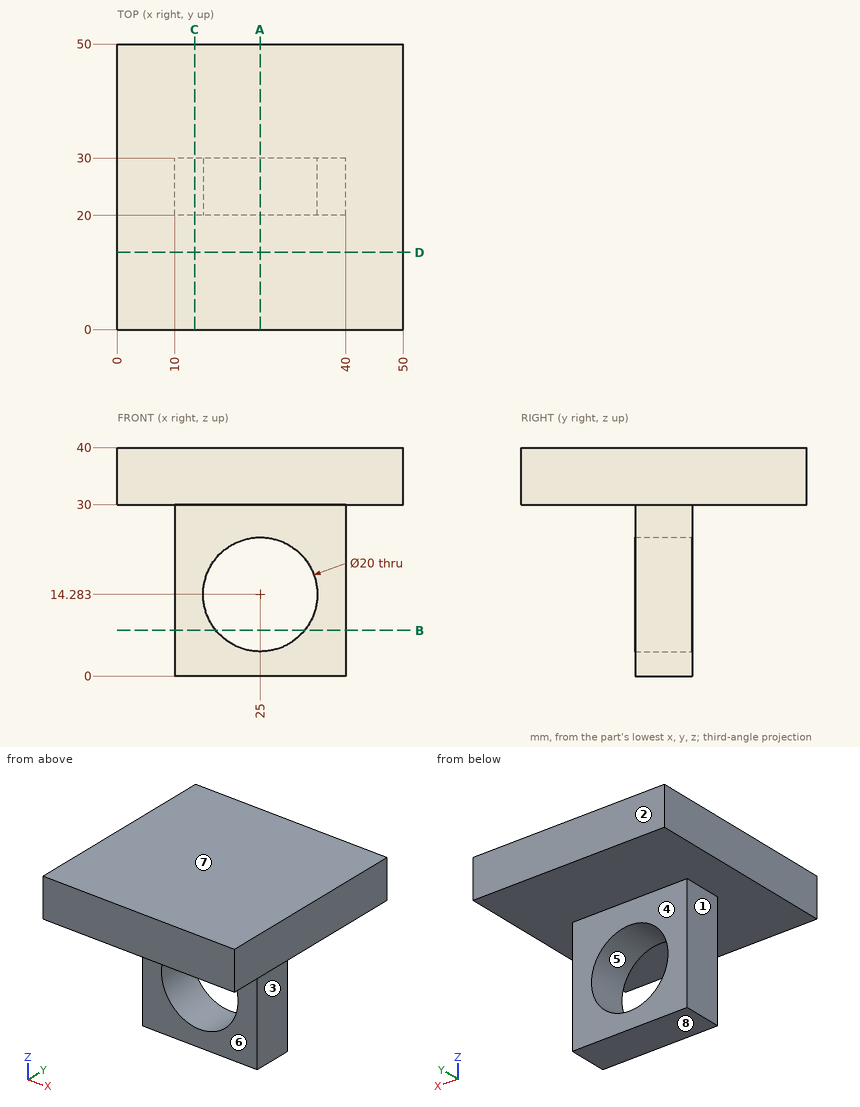
Verification items for this drawing (mm, ordinates from the low corner). A direction names the side the tool comes from. Round coordinates to 2 decimals unless told otherwise and drop trailing zeros. Write each loop counter-clockwise with the first axis right and the second up, starting at its lowest first coordinate (ties: lowest second). Pieces come first, ordered by that corner, then holes. Notation, with made-up numbers: M 3.25,73 L 28.25,73 A29 cw 28.25,97 Z; hole C 22.5,-39 d1. An arc over 180 degrees is marked long. Write item = value, one per line. Start each with the question number.
1. Section check C-C, the plane x = 13.5. Record the cut outline in (y, z).
2. Section check D-D, the plane y = 13.5. Record the cut outline in (x, z), then the cut area to 3 significant figures.
3. Scan lines: line 1 (Z direction, x = 25, y = 25.75); line 2 (Z direction, x = 4, y = 3.5); line 3 (Y direction, x = 37, z = 17.5). Record each from-to range of solid material in increasing order. Write a range as [from, to].
4. Gauge pin test, flat ends, axial feed: pin 1 (2 mm diameter, centred on x = 33.5, y = 7, fed in from -Z); pin 2 (15 mm diameter, centred on x = 18.5, z = 19, fed in from +Y); pin 3 (5 mm diameter, centred on y = 26.5, z = 8.5, fed in from +X). Record the tip position at first contact, or that the pin passes through.
5. Release check for a two-part mould opening along Z. For the marked faces 5, 6, 7 and 8 record: pulls with the +Z half, pulls with the -Z half, needs draft (parallel to the pull), parting line crosses it, or undercut.
6. Tool access check on the marked faces 1, 2, 3 and 4. Record the directions out of +Z, -Z, +X, -X, +Y, -Y that give a thin tool (end or side, any length) a straight path to the whole face; none if there is none.
7. Section check A-A, the plane x = 25. Record the cut outline in (y, z).
8. Section check B-B, the plane z = 8. Record the cut outline in (x, y), then the cut area to 3 significant figures.
Results found:
q1.outline = M 0,30 L 20,30 L 20,0 L 30,0 L 30,30 L 50,30 L 50,40 L 0,40 Z
q2.outline = M 0,30 L 50,30 L 50,40 L 0,40 Z
q2.area = 500 mm^2
q3.line_1 = [0, 4.28], [24.28, 40]
q3.line_2 = [30, 40]
q3.line_3 = [20, 30]
q4.pin_1 = 30
q4.pin_2 = 30
q4.pin_3 = 40
q5.face_5 = undercut
q5.face_6 = needs draft
q5.face_7 = pulls with the +Z half
q5.face_8 = pulls with the -Z half
q6.face_1 = -Z, -X, +Y, -Y
q6.face_2 = +Z, -Z, +X, -X, +Y
q6.face_3 = -Z, +X, +Y, -Y
q6.face_4 = -Z, +X, -X, +Y
q7.outline = M 0,30 L 20,30 L 20,24.28 L 30,24.28 L 30,30 L 50,30 L 50,40 L 0,40 Z; M 20,0 L 30,0 L 30,4.28 L 20,4.28 Z
q8.outline = M 10,20 L 17.22,20 L 17.22,30 L 10,30 Z; M 32.78,20 L 40,20 L 40,30 L 32.78,30 Z
q8.area = 144 mm^2
